CAD build for the part. Positions are in the model's coordinates, mm. A direction names the side the tool comes from. Give positions to 0.01 mm unless a question says otherwise; leave off trailing zeros. Loops run counter-clockwise (first coordinate to the right, second up) from the corner with the lowest first, then second, coordinate; pieces in that order, holes last. Notation, with made-up numbers: (57.25, 36.5) -> (61.25, 36.5) arc R31 ccw to (61.25, 65.5) -> close; hole circle Ø1 at (-12.5, 48). An arc over 180 degrees is marked (long way). Use one line per item in the form item = value.
```python
from build123d import *

# Parameters (mm, degrees)
SKETCH1_W               = 212
SKETCH1_H               = 40
SKETCH1_R               = 4.075
SKETCH1_R_2             = 1.5
SKETCH1_R_3             = 5
BOSS_EXTRUDE1_DEPTH     = 40
CUT_EXTRUDE3_DEPTH      = 116.047816146
CUT_EXTRUDE3_DEPTH_BACK = 116.047816146
SKETCH2_R               = 1.5
SKETCH2_W               = 58
SKETCH2_H               = 70
SKETCH2_W_2             = 40
SKETCH2_H_2             = 65
FILLET1_R               = 5
FILLET2_R               = 5
SKETCH4_R               = 11
CUT_EXTRUDE4_DEPTH      = 37.5
SKETCH5_R               = 3
CUT_EXTRUDE5_DEPTH      = 5


with BuildPart() as part:
    # Sketch1 → Boss-Extrude1 (new, symmetric)
    with BuildSketch(Plane.XY):
        Rectangle(SKETCH1_W, SKETCH1_H)
        with Locations((-96, 0)):
            Circle(SKETCH1_R, mode=Mode.SUBTRACT)
        with Locations((-81, 15.6)):
            Circle(SKETCH1_R_2, mode=Mode.SUBTRACT)
        with Locations((-49.8, 15.6)):
            Circle(SKETCH1_R_2, mode=Mode.SUBTRACT)
        with Locations((-81, -15.6)):
            Circle(SKETCH1_R_2, mode=Mode.SUBTRACT)
        with Locations((-49.8, -15.6)):
            Circle(SKETCH1_R_2, mode=Mode.SUBTRACT)
        with Locations((91, 0)):
            Circle(SKETCH1_R_3, mode=Mode.SUBTRACT)
        with Locations((58, 13)):
            Circle(SKETCH1_R_2, mode=Mode.SUBTRACT)
        with Locations((58, -13)):
            Circle(SKETCH1_R_2, mode=Mode.SUBTRACT)
        with BuildLine():
            Line((-65.4, 11.5), (-57.4, 11.5))
            ThreePointArc((-57.4, 11.5), (-45.9, 0), (-57.4, -11.5))
            Line((-57.4, -11.5), (-65.4, -11.5))
            ThreePointArc((-65.4, -11.5), (-76.9, 0), (-65.4, 11.5))
        make_face(mode=Mode.SUBTRACT)
    extrude(amount=BOSS_EXTRUDE1_DEPTH, both=True)

    # Sketch2 → Cut-Extrude3 (cut, two sides: drawn at the far end of the back side and taken through both)
    with BuildSketch(Plane(origin=(0, 0, 0), x_dir=(1, 0, 0), z_dir=(0, 1, 0)).offset(-CUT_EXTRUDE3_DEPTH_BACK)):
        with Locations(Location((-96, 25, 0), (0, 0, 270))):
            Circle(SKETCH2_R)
        with Locations(Location((-96, -25, 0), (0, 0, 270))):
            Circle(SKETCH2_R)
        with Locations((-58, 0)):
            Rectangle(SKETCH2_W, SKETCH2_H)
        Polygon((-19, 24.740857736), (45.00806186, -35), (-19, -35), align=None)
        with Locations((86, 0)):
            Rectangle(SKETCH2_W_2, SKETCH2_H_2)
        Polygon((-8.00806186, 35), (56, -24.740857736), (56, 35), align=None)
    extrude(amount=CUT_EXTRUDE3_DEPTH + CUT_EXTRUDE3_DEPTH_BACK, mode=Mode.SUBTRACT)

    # Fillet1
    fillet1_edges = [part.edges().sort_by_distance(p)[0] for p in [
        (56, 0, -35),
        (56, 0, 24.740857736),
        (-8.00806186, 0, -35),
        (45.00806186, 0, 35),
        (-19, 0, 35),
        (-19, 0, -24.740857736),
    ]]
    fillet(fillet1_edges, radius=FILLET1_R)

    # Fillet2
    fillet2_edges = [part.edges().sort_by_distance(p)[0] for p in [
        (106, -20, 36.25),
        (-106, -20, 0),
        (-106, 20, 0),
        (106, 20, 36.25),
        (106, -20, -36.25),
        (106, 20, -36.25),
    ]]
    fillet(fillet2_edges, radius=FILLET2_R)

    # Sketch4 → Cut-Extrude4 (cut, symmetric)
    with BuildSketch(Plane.XY):
        with Locations((91, 0)):
            Circle(SKETCH4_R)
    extrude(amount=CUT_EXTRUDE4_DEPTH, both=True, mode=Mode.SUBTRACT)

    # Sketch5 → Cut-Extrude5 (cut)
    with BuildSketch(Plane(origin=(0, 20, 0), x_dir=(1, 0, 0), z_dir=(0, 1, 0))):
        with Locations(Location((-96, 25, 0), (0, 0, 270))):
            Circle(SKETCH5_R)
        with Locations(Location((-96, -25, 0), (0, 0, 270))):
            Circle(SKETCH5_R)
    extrude(amount=-CUT_EXTRUDE5_DEPTH, mode=Mode.SUBTRACT)


solid = part.part
```
1. Cut at A-A, the plane x = -62. Write the cut outline in (y, z).
Result sheet:
outline = (-20, -40) -> (-11.5, -40) -> (-11.5, -35) -> (-20, -35) -> close; (-20, 35) -> (-11.5, 35) -> (-11.5, 40) -> (-20, 40) -> close; (11.5, -40) -> (20, -40) -> (20, -35) -> (11.5, -35) -> close; (11.5, 35) -> (20, 35) -> (20, 40) -> (11.5, 40) -> close
2. Cut at C-C, the plane x = 91. Write the cut outline in (y, z).
Result sheet:
outline = (-20, -40) -> (-5, -40) -> (-5, -37.5) -> (-11, -37.5) -> (-11, -32.5) -> (-20, -32.5) -> close; (-20, 32.5) -> (-11, 32.5) -> (-11, 37.5) -> (-5, 37.5) -> (-5, 40) -> (-20, 40) -> close; (5, -40) -> (20, -40) -> (20, -32.5) -> (11, -32.5) -> (11, -37.5) -> (5, -37.5) -> close; (5, 37.5) -> (11, 37.5) -> (11, 32.5) -> (20, 32.5) -> (20, 40) -> (5, 40) -> close
3. Drop flat-ended pins along their axis: P1, Ø3.5, axis at x = -81, y = 15.6, coming from the +Z side; P2, Ø3, axis at x = -96.5, z = -25.5, coming from the +Y side. Give the stop position or say it passes through.
Result sheet:
P1 = 40
P2 = 15
4. Tool access for faces 4 (the flat face through (106, 0, 36)), 5 (the cylindrical face through (-45.903, 0.253, -37.465)), 6 (the flat face through (93, -5, -37.5)), 7 (the flat face through (66, 0, 0)), 8 (the flat face through (28, 0, -35)): list every direction of +Z, -Z, +X, -X, +Y, -Y with a clear straight run to the whole face (end or side of a thin tool).
Result sheet:
face_4 = +Z, -Z, +X, +Y, -Y
face_5 = +Z, -Z
face_6 = none
face_7 = +X, +Y, -Y
face_8 = +Y, -Y
5. Mould opens along X. For faces 1 (the flat face through (77, 0, -32.5)), 2 (the flat face through (-87, 0, 0)), 3 (the cylindrical face through (104, -19, 36)) say: pulls with the +X half, pulls with the -X half, needs draft (parallel to the pull), parting line crosses it, or undercut.
Result sheet:
face_1 = needs draft
face_2 = undercut
face_3 = pulls with the +X half
6. Cut at B-B, the plane y = 0. State how many separate pieces and enclosed holes the cut face has, then the cut area to 3 significant figures.
Result sheet:
separate_pieces = 5
enclosed_holes = 2
area = 5,380 mm^2
7. Drill centre lines: line 1 (X direction, y = 5.5, z = -30); line 2 (Y direction, x = -81, z = -36.7); line 3 (Z direction, x = -38.5, y = -10.5). Where is each one in solid material? Low to high.
Result sheet:
line_1 = -106 to -87, -29 to -0.32, 56 to 66
line_2 = -20 to -17.1, -14.1 to 14.1, 17.1 to 20
line_3 = -40 to -35, 35 to 40
